Check sheet for the modelled part. Datum: model origin and axes. Units: mm. A direction names the side the tool comes from. Coordinates: 2 decimals unless noted, no trailing zeros. Loops run counter-clockwise (first coordinate to the right, second up) from the corner with the lowest first, then second, coordinate; pieces in that order, holes last.
```python
from build123d import *

# Parameters (mm, degrees)
SKIZZE1_W                       = 8.7
SKIZZE1_H                       = 3.7
AUFSATZ_LINEAR_AUSTRAGEN1_DEPTH = 3.7
VERRUNDUNG1_R                   = 0.1
SKIZZE2_W                       = 1.6
SKIZZE2_H                       = 3.2
SCHNITT_LINEAR_AUSTRAGEN1_DEPTH = 0.4
SKIZZE3_W                       = 1.5
SKIZZE3_H                       = 1.5
AUFSATZ_LINEAR_AUSTRAGEN2_DEPTH = 4
FASE1_SIZE                      = 0.4
SKIZZE4_W                       = 1
SKIZZE4_H                       = 0.5
AUFSATZ_LINEAR_AUSTRAGEN3_DEPTH = 5
VERRUNDUNG2_R                   = 0.5


with BuildPart() as part:
    # Skizze1 → Aufsatz-Linear austragen1 (new body)
    with BuildSketch(Plane(origin=(0, 0, 0), x_dir=(0, 1, 0), z_dir=(0, 0, 1))):
        Rectangle(SKIZZE1_W, SKIZZE1_H)
    extrude(amount=AUFSATZ_LINEAR_AUSTRAGEN1_DEPTH)

    # Verrundung1
    verrundung1_edges = [part.edges().sort_by_distance(p)[0] for p in [
        (0, -4.35, 3.7),
        (1.85, 0, 3.7),
        (0, 4.35, 3.7),
        (1.85, 0, 0),
        (0, -4.35, 0),
        (-1.85, 0, 0),
        (0, 4.35, 0),
        (1.85, 4.35, 1.85),
        (1.85, -4.35, 1.85),
        (-1.85, -4.35, 1.85),
        (-1.85, 4.35, 1.85),
        (-1.85, 0, 3.7),
    ]]
    fillet(verrundung1_edges, radius=VERRUNDUNG1_R)

    # Skizze2 → Schnitt-Linear austragen1 (cut)
    with BuildSketch(Plane.XY.offset(3.7)):
        Rectangle(SKIZZE2_W, SKIZZE2_H)
    extrude(amount=-SCHNITT_LINEAR_AUSTRAGEN1_DEPTH, mode=Mode.SUBTRACT)

    # Skizze3 → Aufsatz-Linear austragen2 (add)
    with BuildSketch(Plane.XY.offset(3.3)):
        with Locations((0, 0.770929874)):
            Rectangle(SKIZZE3_W, SKIZZE3_H)
    extrude(amount=AUFSATZ_LINEAR_AUSTRAGEN2_DEPTH)

    # Fase1
    fase1_edges = [part.edges().sort_by_distance(p)[0] for p in [
        (0.75, 0.770929874, 7.3),
        (0, 1.520929874, 7.3),
        (-0.75, 0.770929874, 7.3),
        (0, 0.020929874, 7.3),
    ]]
    chamfer(fase1_edges, length=FASE1_SIZE)

    # Skizze4 → Aufsatz-Linear austragen3 (add)
    with BuildSketch(Plane(origin=(0, 0, 0), x_dir=(1, 0, 0), z_dir=(0, 0, -1))):
        with Locations((0, 2.835)):
            Rectangle(SKIZZE4_W, SKIZZE4_H)
        Rectangle(SKIZZE4_W, SKIZZE4_H)
        with Locations((0, -2.83)):
            Rectangle(SKIZZE4_W, SKIZZE4_H)
    extrude(amount=AUFSATZ_LINEAR_AUSTRAGEN3_DEPTH)

    # Verrundung2
    verrundung2_edges = [part.edges().sort_by_distance(p)[0] for p in [
        (-0.5, 2.83, -5),
        (0.5, 2.83, -5),
        (-0.5, 0, -5),
        (0.5, 0, -5),
        (-0.5, -2.835, -5),
        (0.5, -2.835, -5),
    ]]
    fillet(verrundung2_edges, radius=VERRUNDUNG2_R - 0.0001)  # a hair under: the kernel refuses the full size


solid = part.part
```
1) Set-up check for faces 4 (the flat face through (0, -3.085, -2)), 5 (the flat face through (0, 3.08, -2)), 6 (the flat face through (0, 2.58, -2)), 7 (the flat face through (1.85, 0, 2)): record each of +Z, -Z, +X, -X, +Y, -Y from which the full face is reachable in a straight line by a thin tool's end or side.
Answer sheet:
face 4: -Z, +X, -X, -Y
face 5: -Z, +X, -X, +Y
face 6: -Z, +X, -X
face 7: +Z, -Z, +X, +Y, -Y
2) Section check B-B on y = 2. Enter the section's corners in (x, z).
Answer sheet:
outline: (-1.85, 0.1) arc R0.1 ccw to (-1.75, 0) - (1.75, 0) arc R0.1 ccw to (1.85, 0.1) - (1.85, 3.6) arc R0.1 ccw to (1.75, 3.7) - (-1.75, 3.7) arc R0.1 ccw to (-1.85, 3.6) - close
3) Section check D-D on y = 0.75. Enter the section's corners in (x, z), plus the area to 3 significant figures.
Answer sheet:
outline: (-1.85, 0.1) arc R0.1 ccw to (-1.75, 0) - (1.75, 0) arc R0.1 ccw to (1.85, 0.1) - (1.85, 3.6) arc R0.1 ccw to (1.75, 3.7) - (0.8, 3.7) - (0.8, 3.3) - (0.75, 3.3) - (0.75, 6.9) - (0.35, 7.3) - (-0.35, 7.3) - (-0.75, 6.9) - (-0.75, 3.3) - (-0.8, 3.3) - (-0.8, 3.7) - (-1.75, 3.7) arc R0.1 ccw to (-1.85, 3.6) - close
area: 18.9 mm2
4) Mould release check, pull along Y, two halves, no side actions. Record for faces 1 (the flat face through (0, -4.35, 2)), 2 (the flat face through (0, 4.35, 2)), 3 (the flat face through (0, -1, 3.3)): +Y half, -Y half, draft (parallel to the pull), parting line (faces both ways), or undercut.
Answer sheet:
face 1: -Y half
face 2: +Y half
face 3: undercut
5) Section check C-C on x = 1.15. Enter the section's corners in (y, z).
Answer sheet:
outline: (-4.35, 0.1) arc R0.1 ccw to (-4.25, 0) - (4.25, 0) arc R0.1 ccw to (4.35, 0.1) - (4.35, 3.6) arc R0.1 ccw to (4.25, 3.7) - (-4.25, 3.7) arc R0.1 ccw to (-4.35, 3.6) - close
6) Section check A-A on z = -3.25. Enter the section's corners in (x, y) (3 decimals), plus the area to 3 significant figures.
Answer sheet:
outline: (-0.5, -3.085) - (0.5, -3.085) - (0.5, -2.585) - (-0.5, -2.585) - close; (-0.5, -0.25) - (0.5, -0.25) - (0.5, 0.25) - (-0.5, 0.25) - close; (-0.5, 2.58) - (0.5, 2.58) - (0.5, 3.08) - (-0.5, 3.08) - close
area: 1.50 mm2
7) Depth check by flat-ended pin: pin 1 (0.5 mm diameter, centred on x = 0, z = -2, fed in from +Y); pin 2 (2 mm diameter, centred on y = 0.5, z = 5.5, fed in from -X); pin 3 (0.8 mm diameter, centred on y = 1, z = 4.5, fed in from +X). Enter the tip coordinate at first touch or a pass-through.
Answer sheet:
pin 1: stops at y = 3.08
pin 2: stops at x = -0.75
pin 3: stops at x = 0.75
8) Scan lines: line 1 (Y direction, x = 0.1, z = -0.5) (3 decimals); line 2 (Y direction, x = 0.25, z = 5); line 3 (Z direction, x = -0.65, y = -0.5). Record each from-to range of solid material in increasing order.
Answer sheet:
line 1: y = -3.085 to -2.585, -0.25 to 0.25, 2.58 to 3.08
line 2: y = 0.02 to 1.52
line 3: z = 0 to 3.3
